from build123d import *

# Parameters (mm, degrees)
SKETCH_R        = 9
SKETCH_R_2      = 1.6
PAD_DEPTH       = 3
SKETCH001_R     = 7.5
SKETCH001_R_2   = 5.1
PAD001_DEPTH    = 12
SKETCH002_W     = 19
SKETCH002_H     = 19
PAD002_DEPTH    = 3
SKETCH003_R     = 1.6
POCKET_DEPTH    = 3.001
SKETCH004_W     = 11
SKETCH004_H     = 8
PAD003_DEPTH    = 3
FILLET_R        = 3.5
SKETCH005_R     = 1.6
POCKET001_DEPTH = 3.001
SKETCH006_R     = 3.5
POCKET002_DEPTH = 12.001
CHAMFER_SIZE    = 1


with BuildPart() as part:
    # Sketch → Pad (new body)
    with BuildSketch(Plane.XY):
        Circle(SKETCH_R)
        Circle(SKETCH_R_2, mode=Mode.SUBTRACT)
    extrude(amount=PAD_DEPTH)

    # Sketch001 (on Face4 of Pad) → Pad001 (join)
    with BuildSketch(Plane.XY.offset(3)):
        Circle(SKETCH001_R)
        Circle(SKETCH001_R_2, mode=Mode.SUBTRACT)
    extrude(amount=PAD001_DEPTH)

    # Sketch002 (on Face2 of Pad001) → Pad002 (join)
    with BuildSketch(Plane(origin=(0, 0, 0), x_dir=(1, 0, 0), z_dir=(0, 0, -1))):
        with Locations((-4.5, -4.5)):
            Rectangle(SKETCH002_W, SKETCH002_H)
    extrude(amount=-PAD002_DEPTH)

    # Sketch003 (on Face10 of Pad002) → Pocket (cut, through all)
    with BuildSketch(Plane.XY.offset(3)):
        Circle(SKETCH003_R)
    extrude(amount=-POCKET_DEPTH, mode=Mode.SUBTRACT)

    # Sketch004 (on Face16 of Pocket) → Pad003 (join)
    with BuildSketch(Plane.XY.offset(3)):
        with Locations((10.5, 0)):
            Rectangle(SKETCH004_W, SKETCH004_H)
    extrude(amount=-PAD003_DEPTH)

    # Fillet
    fillet_edges = [part.edges().sort_by_distance(p)[0] for p in [
        (-14, -5, 1.5),
        (-14, 14, 1.5),
        (5, 14, 1.5),
        (16, 4, 1.5),
        (16, -4, 1.5),
    ]]
    fillet(fillet_edges, radius=FILLET_R)

    # Sketch005 (on Face24 of Fillet) → Pocket001 (cut, through all)
    with BuildSketch(Plane.XY.offset(3)):
        with Locations((0, 10)):
            Circle(SKETCH005_R)
        with Locations((-10, 0)):
            Circle(SKETCH005_R)
        with Locations((10, 0)):
            Circle(SKETCH005_R)
    extrude(amount=-POCKET001_DEPTH, mode=Mode.SUBTRACT)

    # Sketch006 (on Face9 of Pocket001) → Pocket002 (cut, through all)
    with BuildSketch(Plane.XY.offset(3)):
        with Locations((0, 10)):
            Circle(SKETCH006_R)
        with Locations((-10, 0)):
            Circle(SKETCH006_R)
        with Locations((10, 0)):
            Circle(SKETCH006_R)
    extrude(amount=POCKET002_DEPTH, mode=Mode.SUBTRACT)

    # Chamfer
    chamfer_edges = [part.edges().sort_by_distance(p)[0] for p in [
        (-5.1, 0, 15),
    ]]
    chamfer(chamfer_edges, length=CHAMFER_SIZE)


solid = part.part
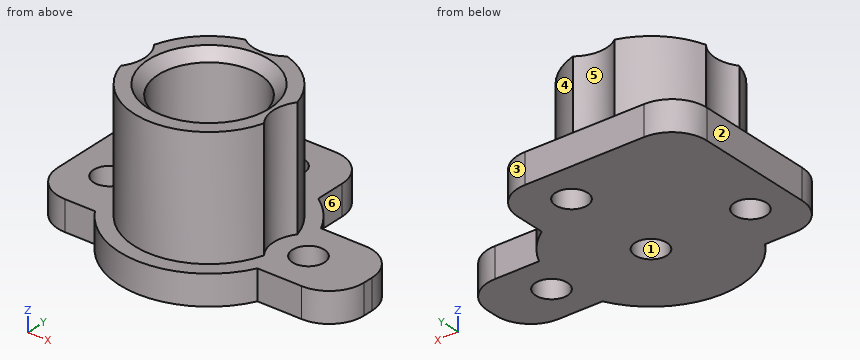
Verification items for the finished model (mm, model axes). Face numbers are marked on the shaded views. A direction names the side the tool comes from. Coordinates: 2 decimals unless noted, no trailing zeros. Order: outer loops, then holes, each group sorted by start corner. A loop starts at its lowest first (then second) coordinate and runs counter-clockwise, first axis right, second up. Notation, with made-up numbers: M 24,56.25 L 62,56.25 A33 cw 62,90.25 Z; hole C 62.25,32.25 d11. An arc over 180 degrees is marked long. One line per item, written item: value. Start each with the question number.
Item 1: Mould release check, pull along Y, two halves, no side actions. Record for the marked faces 1, 2 and 3: released by +Y, released by -Y, zero draft, split by the parting line, or undercut.
Item 2: Gauge pin test, flat ends, axial feed: pin 1 (11 mm diameter, centred on x = 1, y = 0, fed in from +Z); pin 2 (3 mm diameter, centred on x = 0, y = 0, fed in from +Z); pin 3 (8 mm diameter, centred on x = -7.5, z = 7, fed in from -Y); pin 4 (2.5 mm diameter, centred on x = -9.5, z = 1.5, fed in from -Y). Record the tip position at first contact, or that the pin passes through.
Item 3: Sectioned sample at B-B (y = 10). Enter the section's corners in (x, z), then the cut area to 3 significant figures.
Item 4: Sectioned sample at C-C (z = 6.25). Enter the section's corners in (x, y), then the cut area to 3 significant figures.
Item 5: Scan lines: probe 1 along Y at (x, z) = (0, 0.9); probe 2 along Y at (x, z) = (10, 2.05); probe 3 along Z at (x, y) = (3.5, 2.25). Record each from-to range of solid material in increasing order.
Item 6: Access from +Z, -Z, +X, -X, +Y, -Y to the whole of each face (thin tool, end or side, straight path). Record for the marked faces 4, 5 and 6.
Item 7: Sectioned sample at A-A (x = -10). Enter the section's corners in (y, z).
Item 8: Sectioned sample at D-D (y = 0). Enter the section's corners in (x, z).
Conclusion:
1. face 1: undercut
1. face 2: zero draft
1. face 3: released by +Y
2. pin 1: stops at z = 15
2. pin 2: passes through
2. pin 3: stops at y = -6.63
2. pin 4: stops at y = -5
3. outline: M -14,0 L -1.6,0 L -1.6,3 L -14,3 Z; M 1.6,0 L 5,0 L 5,3 L 1.6,3 Z
3. area: 47.4 mm^2
4. outline: M -7.2,-2.1 A7.5 ccw 7.2,-2.1 A3.5 cw 7.2,2.1 A7.5 ccw 2.1,7.2 A3.5 cw -2.1,7.2 A7.5 ccw -7.2,2.1 A3.5 cw Z; hole C 0,0 d10.2
4. area: 86.5 mm^2
5. probe 1: y = -9 to -1.6, 1.6 to 8.4, 11.6 to 14
5. probe 2: y = -4 to -1.6, 1.6 to 4
5. probe 3: z = 0 to 3
6. face 4: +Z, +X, +Y
6. face 5: +Z, +Y
6. face 6: +Z, -Z, +X, +Y
7. outline: M -5,0 L -1.6,0 L -1.6,3 L -5,3 Z; M 1.6,0 L 14,0 L 14,3 L 1.6,3 Z
8. outline: M -14,0 L -11.6,0 L -11.6,3 L -14,3 Z; M -8.4,0 L -1.6,0 L -1.6,3 L -5.1,3 L -5.1,14 L -6.1,15 L -6.5,15 L -6.5,3 L -8.4,3 Z; M 1.6,0 L 8.4,0 L 8.4,3 L 6.5,3 L 6.5,15 L 6.1,15 L 5.1,14 L 5.1,3 L 1.6,3 Z; M 11.6,0 L 16,0 L 16,3 L 11.6,3 Z
